The drawing under review shows one solid part. Ordinate dimensions are in mm from its lowest x, y, z. Coordinates: 2 decimals unless noted, no trailing zeros. Write each loop counter-clockwise with the first axis right and the second up, starting at its lowest first coordinate (ties: lowest second). Pieces come first, ordered by that corner, then holes.
1) Add section A-A, the plane y = 4. State the section outline as (x, z) points.
2) Add section C-C, the plane z = 7. State the section outline as (x, y) points.
3) Mouldability with a two-part tool opening along X and no side actions: class the marked faces 1, 2 and 3 as released by +X, released by -X, zero draft, split by the parting line, or undercut.
4) For line 1 (Y direction, x = 4, z = 11.25); line 2 (X direction, y = 4.25, z = 5); line 3 (Y direction, x = 3.5, z = 2.5), list the stretches that pass through material, from the lowest coordinate up.
5) For P1, Ø3.5, axis at x = 4, y = 4, coming from the +Z side, flat-tipped, find the tip position at first contact; note if it passes through.
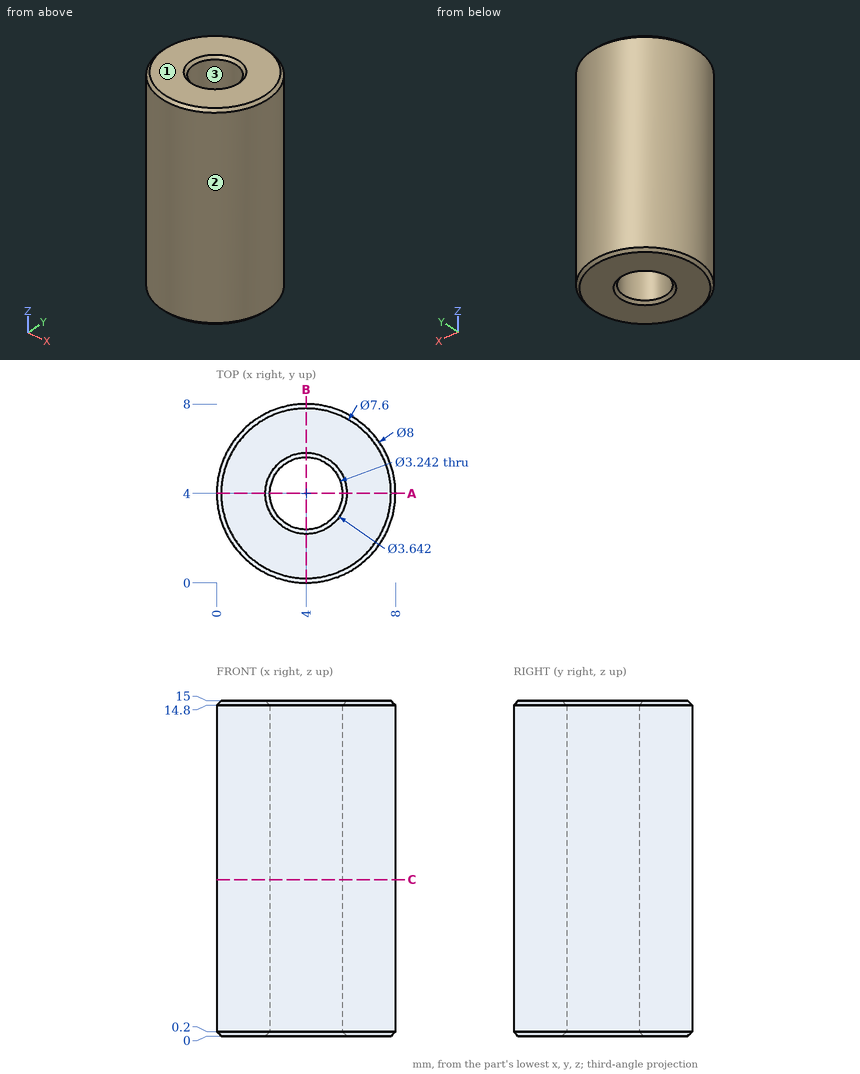
Geometry results:
1. outline: (0, 0.2) - (0.2, 0) - (2.18, 0) - (2.38, 0.2) - (2.38, 14.8) - (2.18, 15) - (0.2, 15) - (0, 14.8) - close; (5.62, 0.2) - (5.82, 0) - (7.8, 0) - (8, 0.2) - (8, 14.8) - (7.8, 15) - (5.82, 15) - (5.62, 14.8) - close
2. outline: circle Ø8 at (4, 4); hole circle Ø3.24 at (4, 4)
3. face 1: zero draft
3. face 2: split by the parting line
3. face 3: undercut
4. line 1: y = 0 to 2.38, 5.62 to 8
4. line 2: x = 0.01 to 2.4, 5.6 to 7.99
4. line 3: y = 0.03 to 2.46, 5.54 to 7.97
5. P1: stops at z = 14.93
